The listing builds one solid part. Answer for the finished solid, in the listing's coordinates (mm). Face numbers are marked on the shaded views. A direction names the side the tool comes from. Round coordinates to 2 decimals unless told otherwise and drop trailing zeros. Order: outer loops, then holes, each group sorted by start corner. A loop starts at its lowest first (then second) coordinate and runs counter-clockwise, first axis right, second up. Notation, with made-up numbers: (50, -35) -> (62, -35) arc R32 ccw to (62, -2) -> close; hole circle Ø11 at (88, -37). An arc over 180 degrees is marked (long way). Answer in a Markdown table with one row per item. Add a question column.
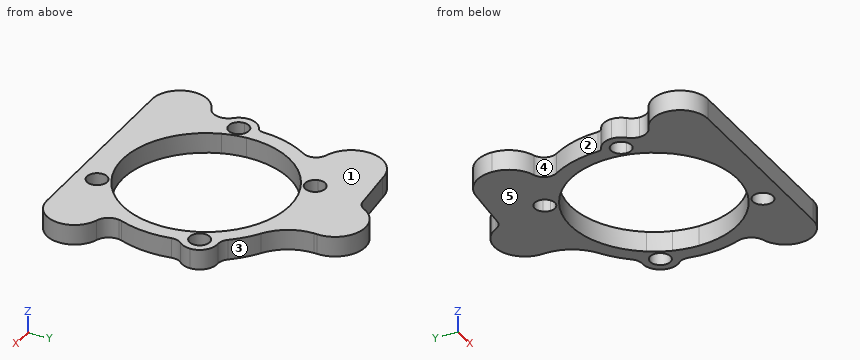
```python
from build123d import *

# Parameters (mm, degrees)
F0_R     = 6.35
F1_DEPTH = 12.7
F2_R     = 7.9375


with BuildPart() as f1:
    # F0 (on Top) → F1 (new body)
    with BuildSketch(Plane.XY):
        with BuildLine():
            ThreePointArc((50.0804162666, 15.375371957), (51.8075185828, 7.7737490661), (52.3875, 0))
            ThreePointArc((52.3875, 0), (8.6161289731, -51.6740987127), (-49.5533247299, -16.9975929021))
            ThreePointArc((-49.5533247299, -16.9975929021), (-51.4249940729, -9.9960062453), (-52.312453003, -2.8031084642))
            ThreePointArc((-52.312453003, -2.8031084642), (-56.8688591942, -0.6489004527), (-61.9082087133, -0.7289376965))
            ThreePointArc((-61.9082087133, -0.7289376965), (-61.8302354833, -3.1905542348), (-61.6544213285, -5.6471220008))
            ThreePointArc((-61.6544213285, -5.6471220008), (-55.692265244, -6.2283994183), (-52.8666598415, -11.5105526461))
            ThreePointArc((-52.8666598415, -11.5105526461), (-59.2166598415, -17.8605526461), (-65.5666598415, -11.5105526461))
            Line((-65.5666598415, -11.5105526461), (-70.3291598415, -11.5105526461))
            ThreePointArc((-70.3291598415, -11.5105526461), (-69.508132002, -15.702599523), (-67.166368927, -19.2752021362))
            ThreePointArc((-67.166368927, -19.2752021362), (-65.1591434342, -22.3374329476), (-64.4554052861, -25.9306159849))
            ThreePointArc((-64.4554052861, -25.9306159849), (-66.044465468, -31.1981091461), (-70.2814387145, -34.7080456373))
            ThreePointArc((-70.2814387145, -34.7080456373), (-80.6164344901, -54.2592739984), (-63.5, -68.2625))
            Line((-63.5, -68.2625), (0, -68.2625))
            Line((0, -68.2625), (58.7375, -68.2625))
            ThreePointArc((58.7375, -68.2625), (75.9947089073, -53.4697653418), (64.0142585669, -34.153837521))
            ThreePointArc((64.0142585669, -34.153837521), (58.7813342607, -30.0675851979), (57.4893859738, -23.5551490588))
            ThreePointArc((57.4893859738, -23.5551490588), (57.686142675, -22.631002937), (57.9734917775, -21.7308975281))
            ThreePointArc((57.9734917775, -21.7308975281), (61.831190131, -3.1719998798), (59.8929243466, 15.6842363367))
            ThreePointArc((59.8929243466, 15.6842363367), (55.0226278067, 14.3874475529), (50.0804162666, 15.375371957))
        make_face()
        with Locations((25.4944466395, -54.673017253)):
            Circle(F0_R, mode=Mode.SUBTRACT)
        with BuildLine():
            ThreePointArc((43.9692893127, 28.4807260018), (47.4791991934, 22.1399141869), (50.0804162666, 15.375371957))
            ThreePointArc((50.0804162666, 15.375371957), (55.0226278067, 14.3874475529), (59.8929243466, 15.6842363367))
            ThreePointArc((59.8929243466, 15.6842363367), (59.2217483156, 18.053868912), (58.456859062, 20.394932823))
            ThreePointArc((58.456859062, 20.394932823), (48.9179628053, 22.8108206775), (53.1987696631, 31.6709419276))
            ThreePointArc((53.1987696631, 31.6709419276), (51.8970719981, 33.7616879655), (50.5132517682, 35.7990090932))
            ThreePointArc((50.5132517682, 35.7990090932), (46.3892876551, 32.9017052551), (43.9692893127, 28.4807260018))
        make_face()
        with BuildLine():
            ThreePointArc((-52.312453003, -2.8031084642), (-16.1886277928, 49.8234732474), (43.9692893127, 28.4807260018))
            ThreePointArc((43.9692893127, 28.4807260018), (46.3892876551, 32.9017052551), (50.5132517682, 35.7990090932))
            ThreePointArc((50.5132517682, 35.7990090932), (52.310310906, 36.3528661823), (54.1750282482, 36.5957827393))
            ThreePointArc((54.1750282482, 36.5957827393), (50.6015982243, 37.2692654479), (47.7034897917, 39.4656143744))
            ThreePointArc((47.7034897917, 39.4656143744), (40.8771414604, 46.4996447543), (33.0262233797, 52.3681795132))
            ThreePointArc((33.0262233797, 52.3681795132), (17.1888443577, 59.4785783783), (-4.35e-08, 61.9125))
            ThreePointArc((-4.35e-08, 61.9125), (-10.3428083822, 61.0424767766), (-20.394932823, 58.456859062))
            ThreePointArc((-20.394932823, 58.456859062), (-19.4651675477, 56.6655768212), (-19.1444466395, 54.673017253))
            ThreePointArc((-19.1444466395, 54.673017253), (-24.7522354429, 48.3665426007), (-31.6709419276, 53.1987696631))
            ThreePointArc((-31.6709419276, 53.1987696631), (-43.3001474916, 44.252173771), (-52.4975053225, 32.8202618997))
            ThreePointArc((-52.4975053225, 32.8202618997), (-59.2888527637, 17.8322627339), (-61.8922171982, 1.5846471339))
            ThreePointArc((-61.8922171982, 1.5846471339), (-62.4517909232, -0.1996749025), (-63.8695481256, -1.4190568766))
            ThreePointArc((-63.8695481256, -1.4190568766), (-68.5759567517, -5.5196247049), (-70.3291598415, -11.5105526461))
            Line((-70.3291598415, -11.5105526461), (-65.5666598415, -11.5105526461))
            ThreePointArc((-65.5666598415, -11.5105526461), (-64.4988130692, -7.9861580486), (-61.6544213285, -5.6471220008))
            ThreePointArc((-61.6544213285, -5.6471220008), (-61.8302354833, -3.1905542348), (-61.9082087133, -0.7289376965))
            ThreePointArc((-61.9082087133, -0.7289376965), (-56.8688591942, -0.6489004527), (-52.312453003, -2.8031084642))
        make_face()
        with BuildLine():
            ThreePointArc((58.456859062, 20.394932823), (59.2217483156, 18.053868912), (59.8929243466, 15.6842363367))
            ThreePointArc((59.8929243466, 15.6842363367), (64.1991359229, 19.7724959812), (65.785517253, 25.4944466395))
            ThreePointArc((65.785517253, 25.4944466395), (62.3526576558, 33.526306918), (54.1750282482, 36.5957827393))
            ThreePointArc((54.1750282482, 36.5957827393), (52.310310906, 36.3528661823), (50.5132517682, 35.7990090932))
            ThreePointArc((50.5132517682, 35.7990090932), (51.8970719981, 33.7616879655), (53.1987696631, 31.6709419276))
            ThreePointArc((53.1987696631, 31.6709419276), (58.6075456748, 30.4786202017), (61.023017253, 25.4944466395))
            ThreePointArc((61.023017253, 25.4944466395), (60.3453137671, 22.6400548906), (58.456859062, 20.394932823))
        make_face()
        with BuildLine():
            ThreePointArc((-4.35e-08, 61.9125), (17.1888443577, 59.4785783783), (33.0262233797, 52.3681795132))
            ThreePointArc((33.0262233797, 52.3681795132), (22.7049210277, 63.3125798927), (18.9534219493, 77.8808823529))
            ThreePointArc((18.9534219493, 77.8808823529), (18.9682238309, 78.8257127153), (19.0126149481, 79.7696157495))
            ThreePointArc((19.0126149481, 79.7696157495), (13.041818397, 67.0767708906), (-4.35e-08, 61.9125))
        make_face()
        with BuildLine():
            ThreePointArc((-20.394932823, 58.456859062), (-10.3428083822, 61.0424767766), (-4.35e-08, 61.9125))
            ThreePointArc((-4.35e-08, 61.9125), (-3.8885649879, 62.3135975568), (-7.6133825433, 63.5))
            Line((-7.6133825433, 63.5), (-50.8, 63.5))
            Line((-50.8, 63.5), (-70.64375, 63.5))
            ThreePointArc((-70.64375, 63.5), (-66.8192563388, 51.788559422), (-56.8199676592, 44.5914198459))
            ThreePointArc((-56.8199676592, 44.5914198459), (-51.7769282768, 39.7640636512), (-52.4975053225, 32.8202618997))
            ThreePointArc((-52.4975053225, 32.8202618997), (-43.3001474916, 44.252173771), (-31.6709419276, 53.1987696631))
            ThreePointArc((-31.6709419276, 53.1987696631), (-28.1780726016, 60.4280717007), (-20.394932823, 58.456859062))
        make_face()
        with BuildLine():
            ThreePointArc((-7.6133825433, 63.5), (-3.8885649879, 62.3135975568), (-4.35e-08, 61.9125))
            ThreePointArc((-4.35e-08, 61.9125), (13.041818397, 67.0767708906), (19.0126149481, 79.7696157495))
            ThreePointArc((19.0126149481, 79.7696157495), (5.2010600776, 99.2887509551), (-16.8048050509, 89.934736466))
            ThreePointArc((-16.8048050509, 89.934736466), (-19.4314787596, 87.050449272), (-23.1150084474, 85.7658729107))
            Line((-23.1150084474, 85.7658729107), (-50.8, 83.34375))
            ThreePointArc((-50.8, 83.34375), (-64.8316501892, 77.5316501892), (-70.64375, 63.5))
            Line((-70.64375, 63.5), (-50.8, 63.5))
            Line((-50.8, 63.5), (-7.6133825433, 63.5))
        make_face()
    extrude(amount=F1_DEPTH)

    # F2
    f2_edges = [f1.edges().sort_by_distance(p)[0] for p in [
        (59.892924, 15.684236, 6.35),
    ]]
    fillet(f2_edges, radius=F2_R)


solid = f1.part
```
1. Straight lines are drawn through the part: line 1 along Y through (x, z) = (-24, 2); line 2 along Y through (x, z) = (26.5, 5.5); line 3 along Y through (x, z) = (54, 3.25). For each, find the intervals that lie inside material, in ascending order.
2. The part is cut by section C-C (x = -27). Give the vertices of the cut face in (y, z), then the cut area to 3 significant figures.
3. The part is cut by section D-D (z = 8.5). Give the number of separate pieces and of enclosed holes in the cut face, then the cut area to 3 significant figures.
4. The mould has two halves that part along Y. Classify the marked faces 3, 4 and 5: released by +Y, released by -Y, zero draft, split by the parting line, or undercut.
5. For the marked faces 1 and 2, determine the directions among +Z, -Z, +X, -X, +Y, -Y from which every point of the face is accessible in a straight line to the end or side of a thin tool.
6. The part is cut by section A-A (x = 1). Give the vertices of the cut face in (y, z), then the cut area to 3 significant figures.
7. Each of these flat-tipped pins is pushed along its axis until it touches: pin 1 (1 mm diameter, centred on x = -23.5, z = 4, fed in from +Y); pin 2 (6 mm diameter, centred on y = -38.5, z = 6, fed in from +X); pin 3 (11.5 mm diameter, centred on x = 54.67, y = 25.49, fed in from +Z); pin 4 (1.5 mm diameter, centred on x = 10, z = 10.5, fed in from +Y). Where does it stop, or does it pass through?
8. The part is cut by section B-B (y = -31). Give the vertices of the cut face in (x, z), then the cut area to 3 significant figures.
Report:
| question | item | result |
|---|---|---|
| 1 | line 1 | y = -68.26 to -46.57, 46.57 to 48.5, 60.84 to 85.69 |
| 1 | line 2 | y = -68.26 to -60.94, -48.4 to -45.19, 45.19 to 57.92 |
| 1 | line 3 | y = -68.26 to 19.18, 31.81 to 36.59 |
| 2 | outline | (-68.26, 0) -> (-44.89, 0) -> (-44.89, 12.7) -> (-68.26, 12.7) -> close; (44.89, 0) -> (48.5, 0) -> (48.5, 12.7) -> (44.89, 12.7) -> close; (60.84, 0) -> (85.43, 0) -> (85.43, 12.7) -> (60.84, 12.7) -> close |
| 2 | area | 655 mm^2 |
| 3 | separate pieces | 1 |
| 3 | enclosed holes | 5 |
| 3 | area | 9,660 mm^2 |
| 4 | face 3 | released by +Y |
| 4 | face 4 | undercut |
| 4 | face 5 | zero draft |
| 5 | face 1 | +Z, +X, -X, +Y, -Y |
| 5 | face 2 | +Z, -Z, -X |
| 6 | outline | (-68.26, 0) -> (-52.38, 0) -> (-52.38, 12.7) -> (-68.26, 12.7) -> close; (52.38, 0) -> (99.99, 0) -> (99.99, 12.7) -> (52.38, 12.7) -> close |
| 6 | area | 806 mm^2 |
| 7 | pin 1 | stops at y = 85.78 |
| 7 | pin 2 | stops at x = 73.52 |
| 7 | pin 3 | passes through |
| 7 | pin 4 | stops at y = 97.62 |
| 8 | outline | (-65.92, 0) -> (-42.23, 0) -> (-42.23, 12.7) -> (-65.92, 12.7) -> close; (42.23, 0) -> (59.44, 0) -> (59.44, 12.7) -> (42.23, 12.7) -> close |
| 8 | area | 519 mm^2 |
